Verification items for the finished model (mm, model axes). A direction names the side the tool comes from. Give positions to 0.01 mm unless a question says otherwise; leave off trailing zeros. Order: outer loops, then holes, each group sorted by start corner. A loop starts at its lowest first (then second) coordinate and runs counter-clockwise, first axis right, second up. Notation, with made-up numbers: (59, 35) -> (99, 35) arc R28 ccw to (99, 60) -> close; hole circle Ø7 at (89, 63.25). An arc over 180 degrees is marked (long way). Return JSON: item names as keys, results as strings. Group by question number.
(1) Release check for a two-part mould opening along Y. For faces 3 (the face through (27, 15, 10)), 4 (the face through (0, 17, 11)), 5 (the face through (-51, 8, 10)), 6 (the face through (51, 8, 10)) record: pulls with the +Y half, pulls with the -Y half, needs draft (parallel to the pull), parting line crosses it, or undercut.
(2) Cross-section at B-B on x = -29. Enter the section's corners in (y, z), then the cut area to 3 significant figures.
(3) Thickness scan on line 1 along X through (y, z) = (5.75, 18.5); line 2 along Z through (x, y) = (11.5, 2); line 3 along X through (y, z) = (20, 9.5). Record the ranges inside material, lowest first.
(4) Cross-section at C-C on x = 24. Enter the section's corners in (y, z).
(5) Tool access check on faces 1 (the face through (-4, 15, 0)), 2 (the face through (24.4, 18.5, 9.9)). Record the directions out of +Z, -Z, +X, -X, +Y, -Y that give a thin tool (end or side, any length) a straight path to the whole face; none if there is none.
(6) Cross-section at A-A on y = 10.75. Enter the section's corners in (x, z), then the cut area to 3 significant figures.
(7) Depth check by flat-ended pin: pin 1 Ø9 at (x, y) = (9, 8) entering from -Z; pin 2 Ø1 at (x, z) = (41.5, 14.5) entering from -Y; pin 3 Ø12 at (x, z) = (5, 19.5) entering from +Y. Enter the tip coordinate at first touch or a pass-through.
from build123d import *

# Parameters (mm, degrees)
F0_W     = 1
F0_H     = 20
F0_W_2   = 100
F1_DEPTH = 22
F2_DEPTH = 13
F3_DEPTH = 3
F5_DEPTH = 23
F4_W     = 5
F4_H     = 3
F6_DEPTH = 20
F7_R     = 0.9999


# Not quite as in the source:
# - a fillet or chamfer is up to 0.001 mm smaller than in the source, because OpenCascade refuses the exact size
# - a feature names something its author has since deleted; it is built from what else it names


with BuildPart() as f1:
    # F0 (on Front) → F1 (new body)
    with BuildSketch(Plane.XZ):
        Polygon((51, 20), (51, 0), (54, 0), (54, 23), (-54, 23), (-54, 0), (-51, 0), (-51, 20), (-50, 20), (50, 20), align=None)
        with Locations((-50.5, 10)):
            Rectangle(F0_W, F0_H)
        with Locations((0, 10)):
            Rectangle(F0_W_2, F0_H)
        with Locations((50.5, 10)):
            Rectangle(F0_W, F0_H)
    extrude(amount=-F1_DEPTH)

    # F0 (on Front) → F2 (cut)
    with BuildSketch(Plane.XZ):
        with Locations((-50.5, 10)):
            Rectangle(F0_W, F0_H)
        with Locations((0, 10)):
            Rectangle(F0_W_2, F0_H)
        with Locations((50.5, 10)):
            Rectangle(F0_W, F0_H)
    extrude(amount=-F2_DEPTH, mode=Mode.SUBTRACT)

    # F0 (on Front) → F3 (join)
    with BuildSketch(Plane.XZ):
        with Locations((-50.5, 10)):
            Rectangle(F0_W, F0_H)
        with Locations((50.5, 10)):
            Rectangle(F0_W, F0_H)
    extrude(amount=-F3_DEPTH)

    # F4 (on face) → F5 (cut, through all)
    with BuildSketch(Plane(origin=(0, 0, 0), x_dir=(1, 0, 0), z_dir=(0, 0, -1))):
        with BuildLine():
            Line((-16.5831239518, -22), (16.5831239518, -22))
            ThreePointArc((16.5831239518, -22), (0, -17), (-16.5831239518, -22))
        make_face()
    extrude(amount=-F5_DEPTH, mode=Mode.SUBTRACT)

    # F4 (on face) → F6 (cut, through all)
    with BuildSketch(Plane(origin=(0, 0, 0), x_dir=(1, 0, 0), z_dir=(0, 0, -1))):
        with Locations((-44.5, -14.5)):
            Rectangle(F4_W, F4_H)
        with Locations((-34.5, -14.5)):
            Rectangle(F4_W, F4_H)
        with Locations((-24.5, -14.5)):
            Rectangle(F4_W, F4_H)
        with Locations((24.5, -14.5)):
            Rectangle(F4_W, F4_H)
        with Locations((34.5, -14.5)):
            Rectangle(F4_W, F4_H)
        with Locations((44.5, -14.5)):
            Rectangle(F4_W, F4_H)
        with BuildLine():
            Line((-42, -16), (-47, -16))
            ThreePointArc((-47, -16), (-44.5, -18.5), (-42, -16))
        make_face()
        with BuildLine():
            Line((-32, -16), (-37, -16))
            ThreePointArc((-37, -16), (-34.5, -18.5), (-32, -16))
        make_face()
        with BuildLine():
            Line((-22, -16), (-27, -16))
            ThreePointArc((-27, -16), (-24.5, -18.5), (-22, -16))
        make_face()
        with BuildLine():
            ThreePointArc((22, -16), (24.5, -18.5), (27, -16))
            Line((27, -16), (22, -16))
        make_face()
        with BuildLine():
            ThreePointArc((32, -16), (34.5, -18.5), (37, -16))
            Line((37, -16), (32, -16))
        make_face()
        with BuildLine():
            ThreePointArc((42, -16), (44.5, -18.5), (47, -16))
            Line((47, -16), (42, -16))
        make_face()
    extrude(amount=-F6_DEPTH, mode=Mode.SUBTRACT)

    # F7 (radius 1 in the source; OpenCascade refuses exactly that, so slightly less here)
    f7_edges = [f1.edges().sort_by_distance(p)[0] for p in [
        (-54, 22, 11.5),
        (54, 22, 11.5),
        (35.291562, 22, 0),
        (-35.291562, 22, 0),
        (54, 11, 0),
        (-54, 11, 0),
        (-54, 11, 23),
        (-35.291562, 22, 23),
        (35.291562, 22, 23),
        (54, 11, 23),
        (-49, 13, 0),
        (-39.5, 13, 0),
        (-29.5, 13, 0),
        (0, 13, 0),
        (29.5, 13, 0),
        (39.5, 13, 0),
        (49, 13, 0),
        (51, 8, 0),
        (-51, 8, 0),
        (-50, 1.5, 0),
        (50, 1.5, 0),
        (0, 17, 23),
        (0, 17, 0),
        (-47, 13, 10),
        (-42, 13, 10),
        (-37, 13, 10),
        (-32, 13, 10),
        (-27, 13, 10),
        (-22, 13, 10),
        (22, 13, 10),
        (27, 13, 10),
        (32, 13, 10),
        (47, 13, 10),
        (42, 13, 10),
        (37, 13, 10),
        (16.583124, 22, 11.5),
        (-16.583124, 22, 11.5),
    ]]
    fillet(f7_edges, radius=F7_R)


solid = f1.part
Verdict:
{
 "1": {"face 3": "needs draft", "face 4": "pulls with the +Y half", "face 5": "undercut", "face 6": "undercut"},
 "2": {"outline": "(0, 20) -> (13, 20) -> (13, 1) arc R1 ccw to (14, 0) -> (21, 0) arc R1 ccw to (22, 1) -> (22, 22) arc R1 ccw to (21, 23) -> (0, 23) -> close", "area": "245 mm²"},
 "3": {"line 1": "-54 to -51, 51 to 54", "line 2": "20 to 23", "line 3": "-54 to -13.08, 13.08 to 54"},
 "4": {"outline": "(0, 20) -> (18.45, 20) -> (18.45, 0) -> (21, 0) arc R1 ccw to (22, 1) -> (22, 22) arc R1 ccw to (21, 23) -> (0, 23) -> close"},
 "5": {"face 1": "-Z, +X, -X, +Y, -Y", "face 2": "-Z, -Y"},
 "6": {"outline": "(-54, 1) arc R1 ccw to (-53, 0) -> (-52, 0) arc R1 ccw to (-51, 1) -> (-51, 20) -> (51, 20) -> (51, 1) arc R1 ccw to (52, 0) -> (53, 0) arc R1 ccw to (54, 1) -> (54, 22) arc R1 ccw to (53, 23) -> (-53, 23) arc R1 ccw to (-54, 22) -> close", "area": "443 mm²"},
 "7": {"pin 1": "z = 20", "pin 2": "y = 13", "pin 3": "y = 19.09"}
}
